Job drawing, mm, ordinate dimensions from the low corner. One solid piece. Give positions to 0.01 mm unless a question says otherwise; leave off trailing zeros. Order: outer loops, then holes, each group sorted by start corner. A loop starts at its lowest first (then second) coordinate and runs counter-clockwise, first axis right, second up. Notation, with made-up numbers: (-8.75, -38) - (13.25, -38) arc R15 cw to (13.25, -19) - close; hole circle Ø4 at (-1, 45.5). An arc over 180 degrees is marked (long way). One line per item, written item: value.
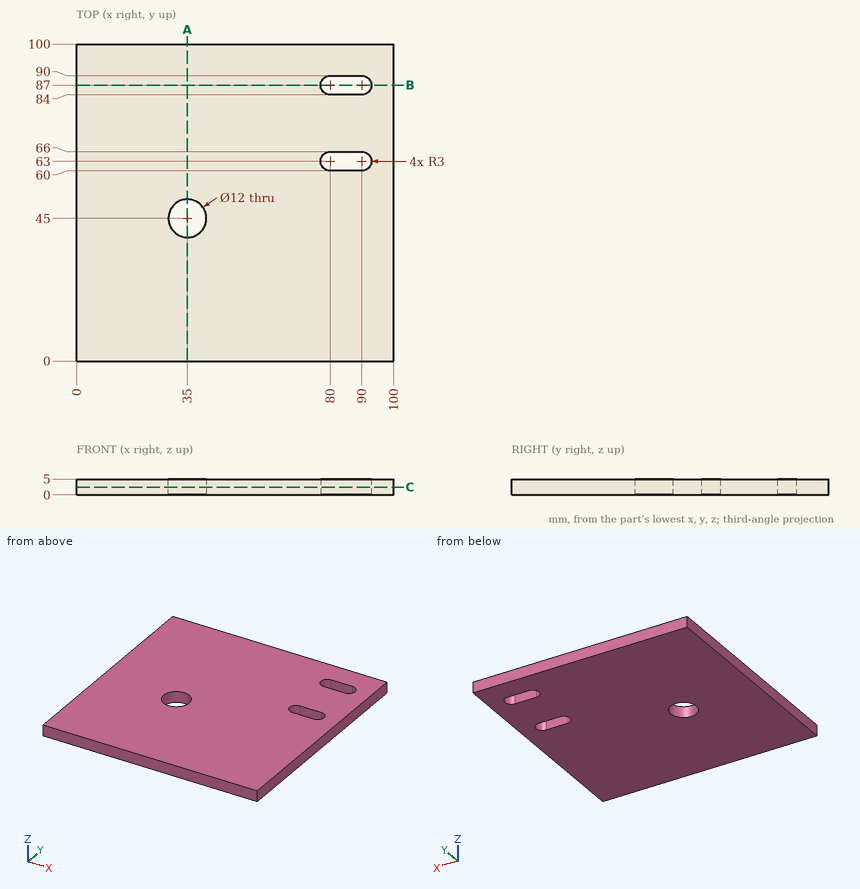
1) Wall check: line 1 along Y through (x, z) = (87, 4.2); line 2 along Y through (x, z) = (35, 2.4); line 3 along X through (y, z) = (40, 4.3). Give the ranges that are in metal, low to high. Write a range as [from, to].
Answer:
line 1: y = [0, 60], [66, 84], [90, 100]
line 2: y = [0, 39], [51, 100]
line 3: x = [0, 31.68], [38.32, 100]
2) Slice it at C-C on z = 2.45. Write the cut outline in (x, y).
Answer:
outline: (0, 0) - (100, 0) - (100, 100) - (0, 100) - close; hole circle Ø12 at (35, 45); hole (80, 60) - (90, 60) arc R3 ccw to (90, 66) - (80, 66) arc R3 ccw to start; hole (80, 84) - (90, 84) arc R3 ccw to (90, 90) - (80, 90) arc R3 ccw to start
3) Slice it at B-B on y = 87. Write the cut outline in (x, z), then the cut area to 3 significant figures.
Answer:
outline: (0, 0) - (77, 0) - (77, 5) - (0, 5) - close; (93, 0) - (100, 0) - (100, 5) - (93, 5) - close
area: 420 mm2
4) Drop a flat-ended pin along its axis: P1, Ø2.5, axis at x = 82.5, z = 3.5, coming from the -Y side. Give the stop position or say it passes through.
Answer:
P1: stops at y = 0
5) Slice it at A-A on x = 35. Write the cut outline in (y, z), then the cut area to 3 significant figures.
Answer:
outline: (0, 0) - (39, 0) - (39, 5) - (0, 5) - close; (51, 0) - (100, 0) - (100, 5) - (51, 5) - close
area: 440 mm2
